Part model, mm, in its own coordinate system. A direction names the side the tool comes from. Give positions to 0.01 mm unless a question says otherwise; leave off trailing zeros. Write each loop counter-clockwise with the first axis right and the second up, starting at its lowest first coordinate (ties: lowest second). Pieces come first, ordered by that corner, then holes. Notation, with made-up numbers: M 69,22.5 L 73,22.5 A19 cw 73,30.5 Z; hole C 55.5,20 d4. An arc over 180 degrees is marked long. Write item = value, one per line. Start each with the question number.
from build123d import *

# Parameters (mm, degrees)
SKETCH_2_R      = 7
SKETCH_2_R_2    = 5
EXTRUDE_1_DEPTH = 2.5
EXTRUDE_START   = -0.5
SKETCH_3_R      = 12
SKETCH_3_R_2    = 7
EXTRUDE_2_DEPTH = 0.5
SKETCH_4_R      = 12
SKETCH_4_R_2    = 7
EXTRUDE_3_DEPTH = 0.5


with BuildPart() as part:
    # 草圖2 → 填料-伸長1 (new body)
    with BuildSketch(Plane(origin=(0, 0, 0), x_dir=(1, 0, 0), z_dir=(0, 1, 0))):
        with Locations(Location((0, 0, 0), (0, 0, 270))):
            Circle(SKETCH_2_R)
        with Locations(Location((0, 0, 0), (0, 0, 270))):
            Circle(SKETCH_2_R_2, mode=Mode.SUBTRACT)
    extrude(amount=EXTRUDE_1_DEPTH)

    # 草圖3 → 填料-伸長2 (add)
    with BuildSketch(Plane(origin=(0, 2.5, 0), x_dir=(1, 0, 0), z_dir=(0, 1, 0)).offset(EXTRUDE_START)):
        with Locations(Location((0, 0, 0), (0, 0, 270))):
            Circle(SKETCH_3_R)
        with Locations(Location((0, 0, 0), (0, 0, 270))):
            Circle(SKETCH_3_R_2, mode=Mode.SUBTRACT)
    extrude(amount=EXTRUDE_2_DEPTH)

    # 草圖4 → 填料-伸長3 (add)
    with BuildSketch(Plane.XZ):
        with Locations(Location((0, 0, 0), (0, 0, 90))):
            Circle(SKETCH_4_R)
        with Locations(Location((0, 0, 0), (0, 0, 270))):
            Circle(SKETCH_4_R_2, mode=Mode.SUBTRACT)
    extrude(amount=-EXTRUDE_3_DEPTH)


solid = part.part
Q1. Two-plate mould, pull along Y, no slides. Class faces 3 (the face through (0.2, 2.5, 5.2)), 4 (the face through (-3.604, 0.246, 11.446)), 5 (the face through (-5.2, 2, 5.2)): +Y half, -Y half, draft (parallel to the pull), parting line (faces both ways), or undercut.
Q2. Slice it at D-D (y = 1.05). Give the cut face in (x, z), and give its area (3 significant figures).
Q3. Tool access for faces 1 (the face through (-6.834, 1.24, -1.517)), 2 (the face through (-0.2, 0, 5.2)): list every direction of +Z, -Z, +X, -X, +Y, -Y with a clear straight run to the whole face (end or side of a thin tool).
Q4. Probe line 1 along Y through (x, z) = (5.25, 7.25); line 2 along X through (y, z) = (1.5, 0); line 3 along Z through (x, y) = (-3.75, 1.45). List the from-to ranges inside material, lowest first.
Q5. Slice it at B-B (x = 0). Give the cut face in (y, z).
Q6. Slice it at C-C (z = 10.25). Give the cut face in (x, y).
Q7. Slice it at A-A (z = 0). Give the cut face in (x, y), and give its area (3 significant figures).
Working result:
q1.face_3 = +Y half
q1.face_4 = draft
q1.face_5 = undercut
q2.outline = C 0,0 d14; hole C 0,0 d10
q2.area = 75.4 mm2
q3.face_1 = none
q3.face_2 = +Z, -Z, +X, -X, -Y
q4.line_1 = 0 to 0.5, 2 to 2.5
q4.line_2 = -7 to -5, 5 to 7
q4.line_3 = -5.91 to -3.31, 3.31 to 5.91
q5.outline = M 0,-12 L 0.5,-12 L 0.5,-7 L 2,-7 L 2,-12 L 2.5,-12 L 2.5,-5 L 0,-5 Z; M 0,5 L 2.5,5 L 2.5,12 L 2,12 L 2,7 L 0.5,7 L 0.5,12 L 0,12 Z
q6.outline = M -6.24,0 L 6.24,0 L 6.24,0.5 L -6.24,0.5 Z; M -6.24,2 L 6.24,2 L 6.24,2.5 L -6.24,2.5 Z
q7.outline = M -12,0 L -5,0 L -5,2.5 L -12,2.5 L -12,2 L -7,2 L -7,0.5 L -12,0.5 Z; M 5,0 L 12,0 L 12,0.5 L 7,0.5 L 7,2 L 12,2 L 12,2.5 L 5,2.5 Z
q7.area = 20.0 mm2
